For this review, take the finished solid that the model builds, in its own axes (mm). A direction names the side the tool comes from. Give positions to 0.01 mm unless a question says otherwise; leave off trailing zeros. Order: outer loops, then holes, each group sorted by start corner. A loop starts at its lowest first (then second) coordinate and runs counter-clockwise, first axis right, second up. Notation, with made-up numbers: (49, 86) -> (101, 86) arc R13 cw to (101, 90) -> close; hole circle Ø11 at (-33.5, 56.5). An arc over 180 degrees is marked (long way). One line per item, written item: value. Start each with the question number.
from build123d import *

# Parameters (mm, degrees)
EXTRUIR_L_MINA1_DEPTH = 230
CROQUIS2_R            = 2
CORTAR_EXTRUIR1_DEPTH = 1
CROQUIS3_W            = 16.026065554
CROQUIS3_H            = 16.026065555
CORTAR_EXTRUIR2_DEPTH = 1


with BuildPart() as part:
    # Croquis1 → Extruir-Lámina1 (new body)
    with BuildSketch(Plane.XY):
        Polygon((-38.118921946, 44.586627311), (-38.118921946, 34.586627311), (-29.118921946, 34.586627311), (-29.118921946, -105.413372689), (-28.118921946, -105.413372689), (-28.118921946, 35.586627311), (-37.118921946, 35.586627311), (-37.118921946, 44.586627311), align=None)
    extrude(amount=EXTRUIR_L_MINA1_DEPTH)

    # Croquis2 → Cortar-Extruir1 (cut)
    with BuildSketch(Plane(origin=(-37.118921946, 0, 0), x_dir=(0, 0, -1), z_dir=(1, 0, 0))):
        with Locations((-190, 39.586627311)):
            Circle(CROQUIS2_R)
        with Locations((-40, 39.586627311)):
            Circle(CROQUIS2_R)
    extrude(amount=-CORTAR_EXTRUIR1_DEPTH, mode=Mode.SUBTRACT)

    # Croquis3 → Cortar-Extruir2 (cut)
    with BuildSketch(Plane(origin=(-28.118921946, 0, 0), x_dir=(0, 0, -1), z_dir=(1, 0, 0))):
        with Locations((-115, -32.426405467)):
            Rectangle(CROQUIS3_W, CROQUIS3_H)
    extrude(amount=-CORTAR_EXTRUIR2_DEPTH, mode=Mode.SUBTRACT)


solid = part.part
Q1. Take a section at A-A (z = 197.5). State the section outline as (x, y) points, and give its area (3 significant figures).
Q2. For faces 1 (the flat face through (-29.119, -19, 113)), 2 (the flat face through (-28.119, -52, 113)), 3 (the flat face through (-33, 35.587, 113)), list the 3-axis set-ups (+Z, -Z, +X, -X, +Y, -Y) from which the entire face can be reached by the end or side of a thin tool; tool diameter is ignored.
Q3. Take a section at B-B (x = -34). State the section outline as (y, z) points.
Q4. For line 1 along Y through (x, z) = (-36.5, 23.5); line 2 along Y through (x, z) = (-37.65, 40); line 3 along X through (y, z) = (-48, 144.5), list the stretches that pass through material, from the lowest coordinate up.
Q5. Take a section at C-C (y = -45). State the section outline as (x, z) points, and give its area (3 significant figures).
Q6. For pin 1 Ø6 at (x, z) = (-34, 112.5) entering from -Y; pin 2 Ø7 at (y, z) = (42, 83) entering from +X; pin 3 Ø12 at (y, z) = (-43, 116) entering from -X; pin 4 Ø4.5 at (y, z) = (39.59, 40) entering from -X, all flat-tipped, find the tip position at first contact; note any pin that passes through.
Answers below:
1. outline: (-38.12, 34.59) -> (-29.12, 34.59) -> (-29.12, -105.41) -> (-28.12, -105.41) -> (-28.12, 35.59) -> (-37.12, 35.59) -> (-37.12, 44.59) -> (-38.12, 44.59) -> close
1. area: 159 mm²
2. face 1: +Z, -Z, -X, -Y
2. face 2: +Z, -Z, +X, +Y, -Y
2. face 3: +Z, -Z, +X, +Y
3. outline: (34.59, 0) -> (35.59, 0) -> (35.59, 230) -> (34.59, 230) -> close
4. line 1: y = 34.59 to 35.59
4. line 2: y = 34.59 to 37.59, 41.59 to 44.59
4. line 3: x = -29.12 to -28.12
5. outline: (-29.12, 0) -> (-28.12, 0) -> (-28.12, 230) -> (-29.12, 230) -> close
5. area: 230 mm²
6. pin 1: stops at y = 34.59
6. pin 2: stops at x = -37.12
6. pin 3: stops at x = -29.12
6. pin 4: stops at x = -38.12
